Work out the finished part from the listing and answer in its coordinate system (mm). Face numbers are marked on the shaded views. A direction names the side the tool comes from. Round coordinates to 2 decimals unless told otherwise and drop trailing zeros. Loops run counter-clockwise (first coordinate to the right, second up) from the corner with the lowest first, then second, coordinate; pieces in that order, holes last.
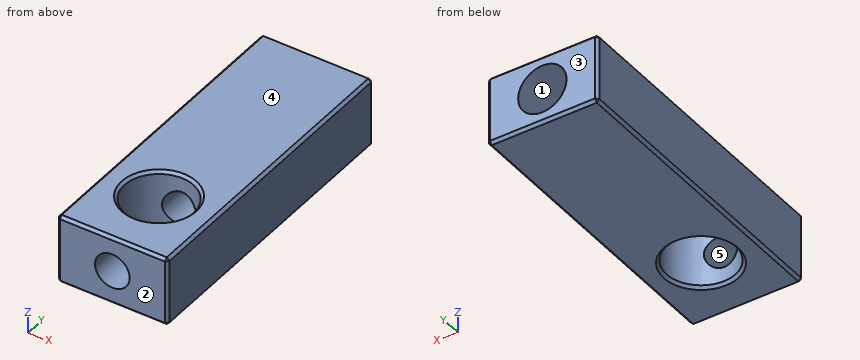
from build123d import *

# Parameters (mm, degrees)
SKIZZE1_W                       = 8
SKIZZE1_H                       = 22
SKIZZE1_R                       = 2.5
AUFSATZ_LINEAR_AUSTRAGEN1_DEPTH = 5
M3_GEWINDEBOHRUNG1_REACH        = 24.913
M3_GEWINDEBOHRUNG1_BORE_R       = 1.25
FASE1_SIZE                      = 0.2
FASE2_SIZE                      = 0.2
SKIZZE4_R                       = 1.75
SCHNITT_LINEAR_AUSTRAGEN1_DEPTH = 13.727922148
M3_GEWINDEBOHRUNG2_D            = 2.5


with BuildPart() as part:
    # Skizze1 → Aufsatz-Linear austragen1 (new body)
    with BuildSketch(Plane.XY):
        with Locations((0, 6)):
            Rectangle(SKIZZE1_W, SKIZZE1_H)
        Circle(SKIZZE1_R, mode=Mode.SUBTRACT)
    extrude(amount=AUFSATZ_LINEAR_AUSTRAGEN1_DEPTH)

    # M3 Gewindebohrung1 bore → M3 Gewindebohrung1 (cut, up to next)
    with BuildSketch(Plane(origin=(0, -5, 0), x_dir=(-1, 0, 0), z_dir=(0, -1, 0)), mode=Mode.PRIVATE) as m3_gewindebohrung1_sk1:
        with Locations((0, -2.5)):
            Circle(M3_GEWINDEBOHRUNG1_BORE_R)
    m3_gewindebohrung1_tool1 = extrude(m3_gewindebohrung1_sk1.sketch, amount=-M3_GEWINDEBOHRUNG1_REACH, mode=Mode.PRIVATE) & part.part
    add(m3_gewindebohrung1_tool1.solids().sort_by_distance((0, -5, 2.5))[0], mode=Mode.SUBTRACT)

    # Fase1
    fase1_edges = [part.edges().sort_by_distance(p)[0] for p in [
        (-2.5, 0, 0),
        (-2.5, 0, 5),
    ]]
    chamfer(fase1_edges, length=FASE1_SIZE)

    # Fase2
    fase2_edges = [part.edges().sort_by_distance(p)[0] for p in [
        (4, 6, 5),
        (0, 17, 5),
        (-4, 6, 5),
        (0, 17, 0),
        (4, 6, 0),
        (0, -5, 0),
        (-4, 6, 0),
        (0, -5, 5),
        (-4, 17, 2.5),
        (4, 17, 2.5),
        (4, -5, 2.5),
        (-4, -5, 2.5),
    ]]
    chamfer(fase2_edges, length=FASE2_SIZE)

    # Skizze4 → Schnitt-Linear austragen1 (cut, through all)
    with BuildSketch(Plane(origin=(0, 6, 0), x_dir=(1, 0, 0), z_dir=(0, 1, 0))):
        with Locations(Location((0, -2.5, 0), (0, 0, 270))):
            Circle(SKIZZE4_R)
    extrude(amount=SCHNITT_LINEAR_AUSTRAGEN1_DEPTH, mode=Mode.SUBTRACT)

    # M3 Gewindebohrung2 (through all)
    with Locations(Plane(origin=(0, 6, 0), x_dir=(1, 0, 0), z_dir=(0, 1, 0))):
        with Locations((0, -2.5)):
            Hole(M3_GEWINDEBOHRUNG2_D / 2)


solid = part.part
Item 1: Section D-D, the plane x = 0 is taken. Give the vertices of the cut face in (y, z), plus the area to 3 significant figures.
Item 2: Section C-C, the plane y = 3.5 is taken. Give the vertices of the cut face in (x, z), plus the area to 3 significant figures.
Item 3: Section A-A, the plane y = 0 is taken. Give the vertices of the cut face in (x, z).
Item 4: Straight lines are drawn through the part: line 1 (Z direction, x = 0, y = -3.8); line 2 (X direction, y = 9.5, z = 2.5); line 3 (Y direction, x = 0, z = 4.3). For each, find the intervals that lie inside material, in ascending order.
Item 5: For the marked faces 1 and 2, determine the directions among +Z, -Z, +X, -X, +Y, -Y from which every point of the face is accessible in a straight line to the end or side of a thin tool.
Item 6: Section B-B, the plane z = 2.5 is taken. Give the vertices of the cut face in (x, y).
Item 7: Determine the mould class of the marked faces 3, 4 and 5 for opening direction Z: pulls with the +Z half, pulls with the -Z half, needs draft (parallel to the pull), parting line crosses it, or undercut.
Answer below:
1. outline: (-5, 0.2) - (-4.8, 0) - (-2.7, 0) - (-2.5, 0.2) - (-2.5, 1.25) - (-5, 1.25) - close; (-5, 3.75) - (-2.5, 3.75) - (-2.5, 4.8) - (-2.7, 5) - (-4.8, 5) - (-5, 4.8) - close; (2.5, 0.2) - (2.7, 0) - (16.8, 0) - (17, 0.2) - (17, 0.75) - (6, 0.75) - (6, 1.25) - (2.5, 1.25) - close; (2.5, 3.75) - (6, 3.75) - (6, 4.25) - (17, 4.25) - (17, 4.8) - (16.8, 5) - (2.7, 5) - (2.5, 4.8) - close
1. area: 31.3 mm2
2. outline: (-4, 0.2) - (-3.8, 0) - (3.8, 0) - (4, 0.2) - (4, 4.8) - (3.8, 5) - (-3.8, 5) - (-4, 4.8) - close; hole circle Ø2.5 at (0, 2.5)
2. area: 35.0 mm2
3. outline: (-4, 0.2) - (-3.8, 0) - (-2.7, 0) - (-2.5, 0.2) - (-2.5, 4.8) - (-2.7, 5) - (-3.8, 5) - (-4, 4.8) - close; (2.5, 0.2) - (2.7, 0) - (3.8, 0) - (4, 0.2) - (4, 4.8) - (3.8, 5) - (2.7, 5) - (2.5, 4.8) - close
4. line 1: z = 0 to 1.25, 3.75 to 5
4. line 2: x = -4 to -1.75, 1.75 to 4
4. line 3: y = -5 to -2.5, 2.5 to 17
5. face 1: +Y
5. face 2: +Z, -Z, +X, -X, -Y
6. outline: (-4, -4.8) - (-3.8, -5) - (-1.25, -5) - (-1.25, -2.17) arc R2.5 cw to (-1.25, 2.17) - (-1.25, 6) - (-1.75, 6) - (-1.75, 17) - (-3.8, 17) - (-4, 16.8) - close; (1.25, -5) - (3.8, -5) - (4, -4.8) - (4, 16.8) - (3.8, 17) - (1.75, 17) - (1.75, 6) - (1.25, 6) - (1.25, 2.17) arc R2.5 cw to (1.25, -2.17) - close
7. face 3: needs draft
7. face 4: pulls with the +Z half
7. face 5: undercut
